Part model, mm, in its own coordinate system. Face numbers are marked on the shaded views. A direction names the side the tool comes from. Coordinates: 2 decimals unless noted, no trailing zeros. Order: outer loops, then holes, each group sorted by start corner. A loop starts at its lowest first (then second) coordinate and runs counter-clockwise, first axis right, second up.
```python
from build123d import *

# Parameters (mm, degrees)
EXTRUDE_1_DEPTH = 10
FILLET_1_R      = 8


with BuildPart() as part:
    # 草图1 → 凸台-拉伸1 (new body)
    with BuildSketch(Plane.XY):
        Polygon((50, 50), (-50, 50), (-50, 42), (-3, 42), (-3, -42), (-50, -42), (-50, -50), (50, -50), (50, -42), (3, -42), (3, 42), (50, 42), align=None)
    extrude(amount=EXTRUDE_1_DEPTH)

    # 圆角1
    fillet_1_edges = [part.edges().sort_by_distance(p)[0] for p in [
        (-3, -42, 5),
        (-3, 42, 5),
        (3, 42, 5),
        (3, -42, 5),
    ]]
    fillet(fillet_1_edges, radius=FILLET_1_R)


solid = part.part
```
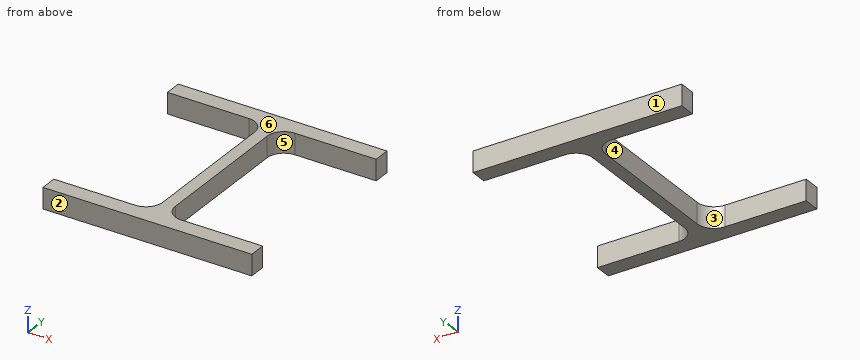
(1) Drop flat-ended pins along their axis: pin 1 (5 mm diameter, centred on y = 5.5, z = 6, fed in from -X); pin 2 (5 mm diameter, centred on y = -13.5, z = 4, fed in from +X); pin 3 (4 mm diameter, centred on x = 12.5, y = -39, fed in from -Z). Give the stop position or say it passes through.
(2) Tool access for the marked faces 4, 5 and 6: list every direction of +Z, -Z, +X, -X, +Y, -Y with a clear straight run to the whole face (end or side of a thin tool).
(3) Slice it at B-B, the plane z = 2.5. Give the cut face in (x, y).
(4) Pull direction Y, two halves, no side cores. Call the marked faces 1, 2 and 3: +Y half, -Y half, draft (parallel to the pull), parting line (faces both ways), or undercut.
(5) Probe line 1 (Y direction, x = -23.5, z = 1); line 2 (X direction, y = -15, z = 1.5); line 3 (X direction, y = 37, z = 1.5). List the from-to ranges inside material, lowest first.
(6) Slice it at C-C, the plane y = -29.5. Give the cut face in (x, z), then the cut area to 3 significant figures.
(7) Slice it at D-D, the plane x = -7. Give the cut face in (y, z), then the cut area to 3 significant figures.
(8) Slice it at A-A, the plane x = 24. Give the cut face in (y, z), then the cut area to 3 significant figures.
Here are the results:
1. pin 1: stops at x = -3
1. pin 2: stops at x = 3
1. pin 3: passes through
2. face 4: +Z, -Z, -X
2. face 5: +Z, -Z, +X
2. face 6: +Z, +X, -X, +Y, -Y
3. outline: (-50, -50) - (50, -50) - (50, -42) - (11, -42) arc R8 cw to (3, -34) - (3, 34) arc R8 cw to (11, 42) - (50, 42) - (50, 50) - (-50, 50) - (-50, 42) - (-11, 42) arc R8 cw to (-3, 34) - (-3, -34) arc R8 cw to (-11, -42) - (-50, -42) - close
4. face 1: +Y half
4. face 2: -Y half
4. face 3: undercut
5. line 1: y = -50 to -42, 42 to 50
5. line 2: x = -3 to 3
5. line 3: x = -3.58 to 3.58
6. outline: (-3, 0) - (3, 0) - (3, 10) - (-3, 10) - close
6. area: 60.0 mm2
7. outline: (-50, 0) - (-40.93, 0) - (-40.93, 10) - (-50, 10) - close; (40.93, 0) - (50, 0) - (50, 10) - (40.93, 10) - close
7. area: 181 mm2
8. outline: (-50, 0) - (-42, 0) - (-42, 10) - (-50, 10) - close; (42, 0) - (50, 0) - (50, 10) - (42, 10) - close
8. area: 160 mm2
